from build123d import *

# Parameters (mm, degrees)
SKETCH1_W           = 47.498
SKETCH1_H           = 12.7
BOSS_EXTRUDE1_DEPTH = 31.75
SKETCH2_R           = 1.4732
CUT_EXTRUDE1_DEPTH  = 47.498
SKETCH3_W           = 19.05
SKETCH3_H           = 8.382
CUT_EXTRUDE2_DEPTH  = 47.498
FILLET1_R           = 5.08
SKETCH4_W           = 47.498
SKETCH4_H           = 4.826
CUT_EXTRUDE3_DEPTH  = 2.54
SKETCH5_W           = 47.498
SKETCH5_H           = 4.826
CUT_EXTRUDE4_DEPTH  = 2.54
SKETCH6_W           = 19.05
SKETCH6_H           = 19.05
CUT_EXTRUDE5_DEPTH  = 2.54
SKETCH7_W           = 19.05
SKETCH7_H           = 17.006147254
CUT_EXTRUDE6_DEPTH  = 2.54
FILLET2_R           = 1.27


with BuildPart() as part:
    # Sketch1 → Boss-Extrude1 (new body)
    with BuildSketch(Plane(origin=(0, 0, 0), x_dir=(1, 0, 0), z_dir=(0, 1, 0))):
        with Locations((23.749, 6.35)):
            Rectangle(SKETCH1_W, SKETCH1_H)
    extrude(amount=BOSS_EXTRUDE1_DEPTH)

    # Sketch2 → Cut-Extrude1 (cut)
    with BuildSketch(Plane.ZY):
        with Locations((-6.35, 3.175)):
            Circle(SKETCH2_R)
        with Locations((-6.35, 28.575)):
            Circle(SKETCH2_R)
    extrude(amount=-CUT_EXTRUDE1_DEPTH, mode=Mode.SUBTRACT)

    # Sketch3 → Cut-Extrude2 (cut)
    with BuildSketch(Plane(origin=(0, 0, -12.7), x_dir=(-1, 0, 0), z_dir=(0, 0, -1))):
        with Locations((-23.749, 4.191)):
            Rectangle(SKETCH3_W, SKETCH3_H)
        with Locations((-23.749, 27.559)):
            Rectangle(SKETCH3_W, SKETCH3_H)
    extrude(amount=-CUT_EXTRUDE2_DEPTH, mode=Mode.SUBTRACT)

    # Fillet1
    fillet1_edges = [part.edges().sort_by_distance(p)[0] for p in [
        (23.749, 8.382, 0),
        (23.749, 8.382, -12.7),
        (23.749, 23.368, 0),
        (23.749, 23.368, -12.7),
    ]]
    fillet(fillet1_edges, radius=FILLET1_R)

    # Sketch4 → Cut-Extrude3 (cut)
    with BuildSketch(Plane.XY):
        with Locations((23.749, 15.875)):
            Rectangle(SKETCH4_W, SKETCH4_H)
    extrude(amount=-CUT_EXTRUDE3_DEPTH, mode=Mode.SUBTRACT)

    # Sketch5 → Cut-Extrude4 (cut)
    with BuildSketch(Plane(origin=(0, 0, -12.7), x_dir=(-1, 0, 0), z_dir=(0, 0, -1))):
        with Locations((-23.749, 15.875)):
            Rectangle(SKETCH5_W, SKETCH5_H)
    extrude(amount=-CUT_EXTRUDE4_DEPTH, mode=Mode.SUBTRACT)

    # Sketch6 → Cut-Extrude5 (cut)
    with BuildSketch(Plane.XY):
        with Locations((23.749, 17.907)):
            Rectangle(SKETCH6_W, SKETCH6_H)
    extrude(amount=-CUT_EXTRUDE5_DEPTH, mode=Mode.SUBTRACT)

    # Sketch7 → Cut-Extrude6 (cut)
    with BuildSketch(Plane(origin=(0, 0, -12.7), x_dir=(-1, 0, 0), z_dir=(0, 0, -1))):
        with Locations((-23.749, 16.885073627)):
            Rectangle(SKETCH7_W, SKETCH7_H)
    extrude(amount=-CUT_EXTRUDE6_DEPTH, mode=Mode.SUBTRACT)

    # Fillet2
    fillet2_edges = [part.edges().sort_by_distance(p)[0] for p in [
        (40.386, 13.462, 0),
        (40.386, 13.462, -2.54),
        (40.386, 18.288, -2.54),
        (40.386, 18.288, 0),
        (7.112, 13.462, 0),
        (7.112, 13.462, -2.54),
        (7.112, 18.288, -2.54),
        (7.112, 18.288, 0),
        (7.112, 31.75, 0),
        (40.386, 31.75, 0),
        (7.112, 0, 0),
        (40.386, 0, 0),
        (40.386, 0, -12.7),
        (40.386, 31.75, -12.7),
        (40.386, 13.462, -12.7),
        (40.386, 13.462, -10.16),
        (40.386, 18.288, -10.16),
        (40.386, 18.288, -12.7),
        (7.112, 31.75, -12.7),
        (7.112, 18.288, -12.7),
        (7.112, 18.288, -10.16),
        (7.112, 0, -12.7),
        (7.112, 13.462, -12.7),
        (7.112, 13.462, -10.16),
    ]]
    fillet(fillet2_edges, radius=FILLET2_R - 0.0001)  # a hair under: the kernel refuses the full size


solid = part.part
Geometry check sheet. Reference: the model listing, model coordinates, mm. A direction names the side the tool comes from. Coordinates: 2 decimals unless noted, no trailing zeros. Order: outer loops, then holes, each group sorted by start corner. A loop starts at its lowest first (then second) coordinate and runs counter-clockwise, first axis right, second up. Notation, with made-up numbers: (-36.75, -2.75) - (9.25, -2.75) arc R16 ccw to (9.25, 10.25) - close; hole circle Ø1 at (13.5, -1). An arc over 180 degrees is marked (long way). One line per item, written item: value.
(1) Thickness scan on probe 1 along Y at (x, z) = (41.5, -6.35); probe 2 along X at (y, z) = (2.5, -11.25); probe 3 along Z at (x, y) = (6, 16). Record the ranges inside material, lowest first. Write a range as from..to.
Data:
probe 1: y = 0..1.7, 4.65..27.1, 30.05..31.75
probe 2: x = 0..14.22, 33.27..47.5
probe 3: z = -10.16..-2.54
(2) Sectioned sample at C-C (x = 15). Enter the section's corners in (y, z), and give its area (3 significant figures).
Data:
outline: (8.38, -7.62) arc R5.08 ccw to (9.06, -10.16) - (22.69, -10.16) arc R5.08 ccw to (23.37, -7.62) - (23.37, -5.08) arc R5.08 ccw to (22.69, -2.54) - (9.06, -2.54) arc R5.08 ccw to (8.38, -5.08) - close
area: 112 mm^2
(3) Access from +Z, -Z, +X, -X, +Y, -Y to the whole of each face (thin tool, end or side, straight path). Record for faces 1 (the face through (40.286, 13.824, -10.542)), 2 (the face through (40.49, 18.67, -0.36)), 3 (the face through (23, 16, -2.54)).
Data:
face 1: -Z, +X, -X
face 2: +Z, +X, -X
face 3: +Z
(4) Depth check by flat-ended pin: pin 1 Ø1 at (x, y) = (13, 13.5) entering from +Z; pin 2 Ø1 at (x, y) = (30.5, 14) entering from +Z; pin 3 Ø6 at (x, z) = (18.5, -5.5) entering from +Y. Enter the tip coordinate at first touch or a pass-through.
Data:
pin 1: stops at z = -0.29
pin 2: stops at z = -2.54
pin 3: stops at y = 23.37
(5) Sectioned sample at D-D (x = 36). Count the separate pieces of the cut face and the enclosed holes in it, and give its area (3 significant figures).
Data:
separate pieces: 1
enclosed holes: 2
area: 364 mm^2
(6) Release check for a two-part mould opening along Y. For faces 4 (the face through (24, 16, -10.16)), 5 (the face through (40, 31.75, -6)), 6 (the face through (23.62, 8.56, -8.95)) record: +Y half, -Y half, draft (parallel to the pull), parting line (faces both ways), or undercut.
Data:
face 4: undercut
face 5: +Y half
face 6: -Y half
(7) Sectioned sample at B-B (y = 10). Enter the section's corners in (x, z), and give its area (3 significant figures).
Data:
outline: (0, -12.7) - (14.22, -12.7) - (14.22, -10.16) - (33.27, -10.16) - (33.27, -12.7) - (47.5, -12.7) - (47.5, 0) - (33.27, 0) - (33.27, -2.54) - (14.22, -2.54) - (14.22, 0) - (0, 0) - close
area: 506 mm^2
(8) Sectioned sample at A-A (z = -6.35). Enter the section's corners in (x, y).
Data:
outline: (0, 0) - (14.22, 0) - (14.22, 1.7) - (0, 1.7) - close; (0, 4.65) - (14.22, 4.65) - (14.22, 8.38) - (33.27, 8.38) - (33.27, 4.65) - (47.5, 4.65) - (47.5, 27.1) - (33.27, 27.1) - (33.27, 23.37) - (14.22, 23.37) - (14.22, 27.1) - (0, 27.1) - close; (0, 30.05) - (14.22, 30.05) - (14.22, 31.75) - (0, 31.75) - close; (33.27, 0) - (47.5, 0) - (47.5, 1.7) - (33.27, 1.7) - close; (33.27, 30.05) - (47.5, 30.05) - (47.5, 31.75) - (33.27, 31.75) - close
